```python
from build123d import *

# Parameters (mm, degrees)
F0_W     = 144.77
F0_H     = 97.62
F1_DEPTH = 150
F2_R     = 5
F3_T     = -1


with BuildPart() as f1:
    # F0 (on Top) → F1 (new body)
    with BuildSketch(Plane.XY):
        Rectangle(F0_W, F0_H)
    extrude(amount=F1_DEPTH)

    # F2
    f2_edges = [f1.edges().sort_by_distance(p)[0] for p in [
        (-72.385, 0, 0),
        (0, -48.81, 0),
        (72.385, 0, 0),
        (0, 48.81, 0),
        (-72.385, -48.81, 75),
        (-72.385, 48.81, 75),
        (72.385, -48.81, 75),
        (72.385, 48.81, 75),
    ]]
    fillet(f2_edges, radius=F2_R)

    # F3
    f3_openings = [f1.faces().sort_by_distance(p)[0] for p in [
        (0, 0, 150),
    ]]
    offset(amount=F3_T, openings=f3_openings)


solid = f1.part
```
The listing builds one solid part. Answer for the finished solid, in the listing's coordinates (mm). A direction names the side the tool comes from. Give positions to 0.01 mm unless a question says otherwise; leave off trailing zeros. Order: outer loops, then holes, each group sorted by start corner. A loop starts at its lowest first (then second) coordinate and runs counter-clockwise, first axis right, second up. Notation, with made-up numbers: M 6,4.5 L 23,4.5 A19 ccw 23,14.5 Z; hole C 87.25,-20 d1. An arc over 180 degrees is marked long. Put each result on its own line as item: value. Start each with the question number.
Item 1: Which of the six approach directions +Z, -Z, +X, -X, +Y, -Y give full straight-line access (tool end or side, diameter ignored) to faces 1 (the face through (-1, 48.81, 76)), 2 (the face through (70.24, 0.61, 2.2))?
Item 2: Find the intervals of material crossed by line 1 along X through (y, z) = (42.5, 118) (3 decimals); line 2 along Y through (x, z) = (-40.5, 60.5); line 3 along Z through (x, y) = (49, 8), in increasing order.
Item 3: The part is cut by section B-B, the plane x = -47. Determine the outline of the cut face in (y, z), and give its area (3 significant figures).
Item 4: The part is cut by section C-C, the plane y = 9.5. Determine the outline of the cut face in (x, z) (3 decimals).
Item 5: For a pull along X with two mould halves and no side action, classify faces 3 (the face through (70.959, 0.613, 1.504)), 4 (the face through (-72.385, -1, 76)), 5 (the face through (-1, 1, 0)), 6 (the face through (-71.385, -1, 76)) as +X half, -X half, draft (parallel to the pull), parting line (faces both ways), or undercut.
Item 6: The part is cut by section A-A, the plane z = 135. Determine the outline of the cut face in (x, y) (3 decimals).
Answer key:
1. face 1: +Z, -Z, +X, -X, +Y
1. face 2: +Z
2. line 1: x = -72.385 to -71.385, 71.385 to 72.385
2. line 2: y = -48.81 to -47.81, 47.81 to 48.81
2. line 3: z = 0 to 1
3. outline: M -48.81,5 A5 ccw -43.81,0 L 43.81,0 A5 ccw 48.81,5 L 48.81,150 L 47.81,150 L 47.81,5 A4 cw 43.81,1 L -43.81,1 A4 cw -47.81,5 L -47.81,150 L -48.81,150 Z
3. area: 392 mm²
4. outline: M -72.385,5 A5 ccw -67.385,0 L 67.385,0 A5 ccw 72.385,5 L 72.385,150 L 71.385,150 L 71.385,5 A4 cw 67.385,1 L -67.385,1 A4 cw -71.385,5 L -71.385,150 L -72.385,150 Z
5. face 3: +X half
5. face 4: -X half
5. face 5: draft
5. face 6: undercut
6. outline: M -72.385,-43.81 A5 ccw -67.385,-48.81 L 67.385,-48.81 A5 ccw 72.385,-43.81 L 72.385,43.81 A5 ccw 67.385,48.81 L -67.385,48.81 A5 ccw -72.385,43.81 Z; hole M -71.385,-43.81 A4 ccw -67.385,-47.81 L 67.385,-47.81 A4 ccw 71.385,-43.81 L 71.385,43.81 A4 ccw 67.385,47.81 L -67.385,47.81 A4 ccw -71.385,43.81 Z
